Read the model definition and answer for the solid it produces. Units are mm, in the model's axes. Coordinates: 2 decimals unless noted, no trailing zeros. Loops run counter-clockwise (first coordinate to the right, second up) from the corner with the lowest first, then second, coordinate; pieces in that order, holes last. Notation, with made-up numbers: (-7.75, 66) -> (33.25, 66) arc R7 ccw to (33.25, 71) -> close; hole circle Ø6 at (19.5, 75.5). An arc over 180 degrees is marked (long way). Answer in a Markdown table with one row per item.
```python
from build123d import *

# Parameters (mm, degrees)
F0_R     = 2.9337
F1_DEPTH = 95.25


with BuildPart() as f1:
    # F0 (on Front) → F1 (new body)
    with BuildSketch(Plane.XZ):
        with BuildLine():
            ThreePointArc((4.818488, -3.645982), (4.237422, -1.477417), (6.405988, -0.896352))
            Line((6.405988, -0.896352), (7.445324, 0.903833))
            Line((7.445324, 0.903833), (6.405987, 2.704018))
            ThreePointArc((6.405987, 2.704018), (4.237422, 3.285083), (4.818487, 5.453648))
            Line((4.818487, 5.453648), (3.77915, 7.253833))
            Line((3.77915, 7.253833), (1.700476, 7.253833))
            ThreePointArc((1.700476, 7.253833), (0.112976, 5.666333), (-1.474524, 7.253833))
            Line((-1.474524, 7.253833), (-3.553199, 7.253832))
            Line((-3.553199, 7.253832), (-4.592536, 5.453648))
            ThreePointArc((-4.592536, 5.453648), (-4.01147, 3.285082), (-6.180035, 2.704017))
            Line((-6.180035, 2.704017), (-7.219372, 0.903832))
            Line((-7.219372, 0.903832), (-6.180035, -0.896352))
            ThreePointArc((-6.180035, -0.896352), (-4.01147, -1.477418), (-4.592535, -3.645983))
            Line((-4.592535, -3.645983), (-3.553198, -5.446168))
            Line((-3.553198, -5.446168), (-1.474524, -5.446167))
            ThreePointArc((-1.474524, -5.446167), (0.112976, -3.858667), (1.700476, -5.446167))
            Line((1.700476, -5.446167), (3.779151, -5.446167))
            Line((3.779151, -5.446167), (4.818488, -3.645982))
        make_face()
        with Locations((0.112976, 0.903833)):
            Circle(F0_R, mode=Mode.SUBTRACT)
    extrude(amount=F1_DEPTH)


solid = f1.part
```
1. Given pin 1 Ø1.5 at (x, y) = (-4.5, -15) entering from -Z; pin 2 Ø1.5 at (y, z) = (-65.5, 5) entering from +X; pin 3 Ø3 at (y, z) = (-10.5, -3.5) entering from -X, each flat-ended and moving along its own axis, determine where each tip first touches the part or whether it passes through.
A:
| item | result |
|---|---|
| pin 1 | stops at z = -5.11 |
| pin 2 | stops at x = 4.82 |
| pin 3 | stops at x = -4.59 |
2. A cutting plane is placed at B-B on y = -76. Give the vertices of the cut face in (x, z) (1 decimal), and give its area (3 significant figures).
A:
| item | result |
|---|---|
| outline | (-7.2, 0.9) -> (-6.2, -0.9) arc R1.6 cw to (-4.6, -3.6) -> (-3.6, -5.4) -> (-1.5, -5.4) arc R1.6 cw to (1.7, -5.4) -> (3.8, -5.4) -> (4.8, -3.6) arc R1.6 cw to (6.4, -0.9) -> (7.4, 0.9) -> (6.4, 2.7) arc R1.6 cw to (4.8, 5.5) -> (3.8, 7.3) -> (1.7, 7.3) arc R1.6 cw to (-1.5, 7.3) -> (-3.6, 7.3) -> (-4.6, 5.5) arc R1.6 cw to (-6.2, 2.7) -> close; hole circle Ø5.9 at (0.1, 0.9) |
| area | 88.9 mm2 |
3. A cutting plane is placed at A-A on x = 0.5. Give the vertices of the cut face in (y, z), and give its area (3 significant figures).
A:
| item | result |
|---|---|
| outline | (-95.25, -3.91) -> (0, -3.91) -> (0, -2) -> (-95.25, -2) -> close; (-95.25, 3.81) -> (0, 3.81) -> (0, 5.71) -> (-95.25, 5.71) -> close |
| area | 362 mm2 |
4. The mould has two halves that part along X. Classify faces 1 (the flat face through (4.29, -46.96, -4.56)), 2 (the cylindrical face through (0.148, -46.958, 5.667)), 3 (the cylindrical face through (-0.52, -46.96, -1.96)), 4 (the flat face through (-4.066, -46.958, 6.366)): pulls with the +X half, pulls with the -X half, needs draft (parallel to the pull), parting line crosses it, or undercut.
A:
| item | result |
|---|---|
| face 1 | pulls with the +X half |
| face 2 | undercut |
| face 3 | undercut |
| face 4 | pulls with the -X half |
5. Find the intervals of material crossed by probe 1 along Z at (x, y) = (4.75, -35); probe 2 along Z at (x, y) = (-4, -85.5); probe 3 along Z at (x, y) = (1, -46.5), in increasing order.
A:
| item | result |
|---|---|
| probe 1 | z = -3.76 to -3.6, -0.94 to 2.75, 5.41 to 5.57 |
| probe 2 | z = -4.67 to -3.04, -1.5 to 3.31, 4.85 to 6.48 |
| probe 3 | z = -4.13 to -1.89, 3.7 to 5.94 |
